Source: CAD feature listing. Evaluate the final solid. Frame: model axes, mm. A direction names the side the tool comes from. Give positions to 0.01 mm unless a question says otherwise; leave off trailing zeros. Order: outer loops, then holes, each group sorted by start corner. A loop starts at its lowest first (then second) coordinate and runs counter-clockwise, first axis right, second up. Notation, with made-up numbers: (1.5, 49.5) -> (37.5, 49.5) arc R18 cw to (37.5, 76.5) -> close; hole circle Ø8 at (32.5, 12.25). An arc over 180 degrees is marked (long way). Use CSV: the item, a comma, the result in double quotes.
```python
from build123d import *

# Parameters (mm, degrees)
EXTRU_MINCE1_DEPTH      = 32
ESQUISSE2_R             = 4
ESQUISSE2_R_2           = 1.2
BOSS_EXTRU_1_DEPTH      = 32
CONG_1_R                = 3
ESQUISSE3_R             = 1.5
ENL_V_MAT_EXTRU_1_DEPTH = 89.126236015


with BuildPart() as part:
    # Esquisse1 → Extru.-Mince1 (new body)
    with BuildSketch(Plane(origin=(0, 0, 0), x_dir=(1, 0, 0), z_dir=(0, 1, 0))):
        with BuildLine():
            Line((0, 0), (-60, 0))
            ThreePointArc((-60, 0), (-70.352761804, -1.362966948), (-80, -5.358983849))
            Line((-80, -5.358983849), (-88.038475773, -10))
            Line((-88.038475773, -10), (-89.038475773, -8.267949192))
            Line((-89.038475773, -8.267949192), (-81, -3.626933041))
            ThreePointArc((-81, -3.626933041), (-70.870399894, 0.568884704), (-60, 2))
            Line((-60, 2), (0, 2))
            Line((0, 2), (0, 0))
        make_face()
    extrude(amount=EXTRU_MINCE1_DEPTH)

    # Esquisse2 → Boss.-Extru.1 (add)
    with BuildSketch(Plane(origin=(0, 0, 0), x_dir=(1, 0, 0), z_dir=(0, 1, 0))):
        with Locations((-70, 3)):
            Circle(ESQUISSE2_R)
        with Locations(Location((-70, 3, 0), (0, 0, 270))):
            Circle(ESQUISSE2_R_2, mode=Mode.SUBTRACT)
    extrude(amount=BOSS_EXTRU_1_DEPTH)

    # Congé1
    cong_1_edges = [part.edges().sort_by_distance(p)[0] for p in [
        (-66.28080804, 16, -1.52771906),
        (-72.687893858, 16, -0.037699103),
    ]]
    fillet(cong_1_edges, radius=CONG_1_R)

    # Esquisse3 → Enlèv. mat.-Extru.1 (cut, through all)
    with BuildSketch(Plane(origin=(-17.679491924, 0, -30.621778265), x_dir=(0.8660254037844379, 0, -0.5000000000000014), z_dir=(0.5000000000000014, 0, 0.8660254037844379))):
        with Locations((-77.74355653, 16)):
            Circle(ESQUISSE3_R)
    extrude(amount=-ENL_V_MAT_EXTRU_1_DEPTH, mode=Mode.SUBTRACT)

    # Symétrie1: part across plane


with BuildPart() as part_1:
    add(part.part)
    add(part.part.mirror(Plane(origin=(0, 32, -2), x_dir=(0, 0, 1), z_dir=(1, 0, 0))))


solid = part_1.part
```
1. Ray query, line 1 along X through (y, z) = (20.5, -3); line 2 along X through (y, z) = (6, -4); line 3 along Z through (x, y) = (-70, 17). Return the intervals inside material, ascending.
Answer below:
line 1,"x = -74 to -71.2, -68.8 to -65.59, 65.59 to 68.8, 71.2 to 74"
line 2,"x = -73.87 to -70.66, -69.34 to -66.13, 66.13 to 69.34, 70.66 to 73.87"
line 3,"z = -7 to -4.2, -1.8 to 1.27"
2. Mould query, pull axis X, two halves, no side actions, for faces 1 (the flat face through (84.182, 15.776, 5.464)), 2 (the flat face through (0, 32, -1)), 3 (the cylindrical face through (70.211, 15.776, 1.325)). Classes: released by +X, released by -X, zero draft, split by the parting line, or undercut.
Answer below:
face 1,"released by +X"
face 2,"zero draft"
face 3,"undercut"
3. Pin query (flat end, axial travel): P1, Ø9.5, axis at x = 13, y = 21.5, coming from the +Z side; P2, Ø3, axis at x = -62, y = 14.5, coming from the +Z side; P3, Ø5, axis at y = 13.5, z = 4, coming from the +X side; P4, Ø4, axis at x = 65, z = 3, coming from the -Y side. Return the tip coordinate at first contact, or that it passes through.
Answer below:
P1,"stops at z = 0"
P2,"stops at z = 0.15"
P3,"stops at x = 85.98"
P4,"passes through"
4. Access query for faces 4 (the flat face through (-83.07, 15.78, 7.13)), 5 (the cylindrical face through (-78.459, 15.776, 2.274)), 6 (the cylindrical face through (61.54, 15.78, -1.97)). Directions: +Z, -Z, +X, -X, +Y, -Y. A direction counts if a zero-diameter tool reaches every point of the face in a straight line with its end or side. Return the directions, or none.
Answer below:
face 4,"+Z, +Y, -Y"
face 5,"-Z, -X, +Y, -Y"
face 6,"-Z, +Y, -Y"
5. Section query A-A on x = 37.5. Return loops of the section in (y, z), plus the area to 3 significant figures.
Answer below:
outline,"(0, -2) -> (32, -2) -> (32, 0) -> (0, 0) -> close"
area,"64.0 mm²"
6. Section query B-B on y = 28. Count the separate pieces of the cut face and the enclosed holes in it, plus the area to 3 significant figures.
Answer below:
separate pieces,"1"
enclosed holes,"2"
area,"445 mm²"
